```python
from build123d import *

# Parameters (mm, degrees)
SKETCH1_R           = 1.25
BOSS_EXTRUDE1_DEPTH = 3
FILLET1_R           = 3
FILLET2_R           = 2


with BuildPart() as part:
    # Sketch1 → Boss-Extrude1 (new body)
    with BuildSketch(Plane.XY):
        with BuildLine():
            Line((-0.215618695, 4.237158078), (-12.280236844, -9.121172241))
            ThreePointArc((-12.280236844, -9.121172241), (-12.064618149, -13.358330319), (-7.827460071, -13.142711624))
            Line((-7.827460071, -13.142711624), (0.215618695, -4.237158078))
            Line((0.215618695, -4.237158078), (7.885671037, -11.391188631))
            ThreePointArc((7.885671037, -11.391188631), (11.979783579, -9.716132772), (11.163266713, -5.368619707))
            Line((11.163266713, -5.368619707), (-0.215618695, 4.237158078))
        make_face()
        with Locations((-10.053848457, -11.131941933)):
            Circle(SKETCH1_R, mode=Mode.SUBTRACT)
        with Locations((8.905553546, -8.043078766)):
            Circle(SKETCH1_R, mode=Mode.SUBTRACT)
    extrude(amount=BOSS_EXTRUDE1_DEPTH)

    # Fillet1
    fillet1_edges = [part.edges().sort_by_distance(p)[0] for p in [
        (-0.215618695, 4.237158078, 1.5),
    ]]
    fillet(fillet1_edges, radius=FILLET1_R)

    # Fillet2
    fillet2_edges = [part.edges().sort_by_distance(p)[0] for p in [
        (0.215618695, -4.237158078, 1.5),
    ]]
    fillet(fillet2_edges, radius=FILLET2_R)


solid = part.part
```
The listing builds one solid part. Answer for the finished solid, in the listing's coordinates (mm). A direction names the side the tool comes from. Give positions to 0.01 mm unless a question says otherwise; leave off trailing zeros. Write each loop counter-clockwise with the first axis right and the second up, starting at its lowest first coordinate (ties: lowest second). Pieces come first, ordered by that corner, then holes. Notation, with made-up numbers: (80, -3.75) -> (123, -3.75) arc R31 cw to (123, 32.25) -> close; hole circle Ø7 at (-36, 81). An arc over 180 degrees is marked (long way). Write item = value, one per line. Start each with the question number.
1) Determine the mould class of faces 1 (the face through (0.23, -5.09, 1.52)), 2 (the face through (-0.169, 3.064, 1.521)), 3 (the face through (6.65, -1.56, 1.48)) for opening direction X: +X half, -X half, draft (parallel to the pull), parting line (faces both ways), or undercut.
2) This flat-tipped pin is pushed along its axis until it touches: pin 1 (1.5 mm diameter, centred on x = -3.5, z = 1.5, fed in from -Y). Where does it stop, or does it pass through?
3) The part is cut by section A-A, the plane x = -9.5. Determine the outline of the cut face in (y, z), and give its area (3 significant figures).
4) Which of the six approach directions +Z, -Z, +X, -X, +Y, -Y give full straight-line access (tool end or side, diameter ignored) to faces 4 (the face through (-4.534, -9.496, 1.479)), 5 (the face through (-1, -3, 0))?
5) Straight lines are drawn through the part: line 1 along X through (y, z) = (-8.5, 1.3); line 2 along X through (y, z) = (-9.5, 1.5); line 3 along X through (y, z) = (-10.5, 2.1). For each, find the intervals that lie inside material, in ascending order.
6) The part is cut by section B-B, the plane y = -6.5. Determine the outline of the cut face in (x, z).
7) The part is cut by section C-C, the plane y = -10.75. Determine the outline of the cut face in (x, z), and give its area (3 significant figures).
8) The part is cut by section D-D, the plane z = 1.95. Determine the outline of the cut face in (x, y).
Solutions:
q1.face_1 = undercut
q1.face_2 = parting line
q1.face_3 = +X half
q2.pin_1 = -9.18
q3.outline = (-14.08, 0) -> (-12.25, 0) -> (-12.25, 3) -> (-14.08, 3) -> close; (-10.01, 0) -> (-6.04, 0) -> (-6.04, 3) -> (-10.01, 3) -> close
q3.area = 17.4 mm²
q4.face_4 = +Z, -Z, -Y
q4.face_5 = -Z, +X, -X, +Y, -Y
q5.line_1 = -11.72 to -3.63, 4.79 to 7.74, 10.07 to 12.38
q5.line_2 = -12.57 to -4.54, 5.86 to 12.09
q5.line_3 = -12.99 to -11.13, -8.98 to -5.44, 6.93 to 11.4
q6.outline = (-9.91, 0) -> (-1.83, 0) -> (-1.83, 3) -> (-9.91, 3) -> close; (2.64, 0) -> (12.05, 0) -> (12.05, 3) -> (2.64, 3) -> close
q7.outline = (-13.03, 0) -> (-11.24, 0) -> (-11.24, 3) -> (-13.03, 3) -> close; (-8.86, 0) -> (-5.67, 0) -> (-5.67, 3) -> (-8.86, 3) -> close; (7.2, 0) -> (11.12, 0) -> (11.12, 3) -> (7.2, 3) -> close
q7.area = 26.7 mm²
q8.outline = (-12.28, -9.12) arc R3 ccw to (-7.83, -13.14) -> (-1.15, -5.75) arc R2 cw to (1.7, -5.62) -> (7.89, -11.39) arc R3.5 ccw to (11.16, -5.37) -> (2, 2.37) arc R3 ccw to (-2.16, 2.08) -> close; hole circle Ø2.5 at (-10.05, -11.13); hole circle Ø2.5 at (8.91, -8.04)
